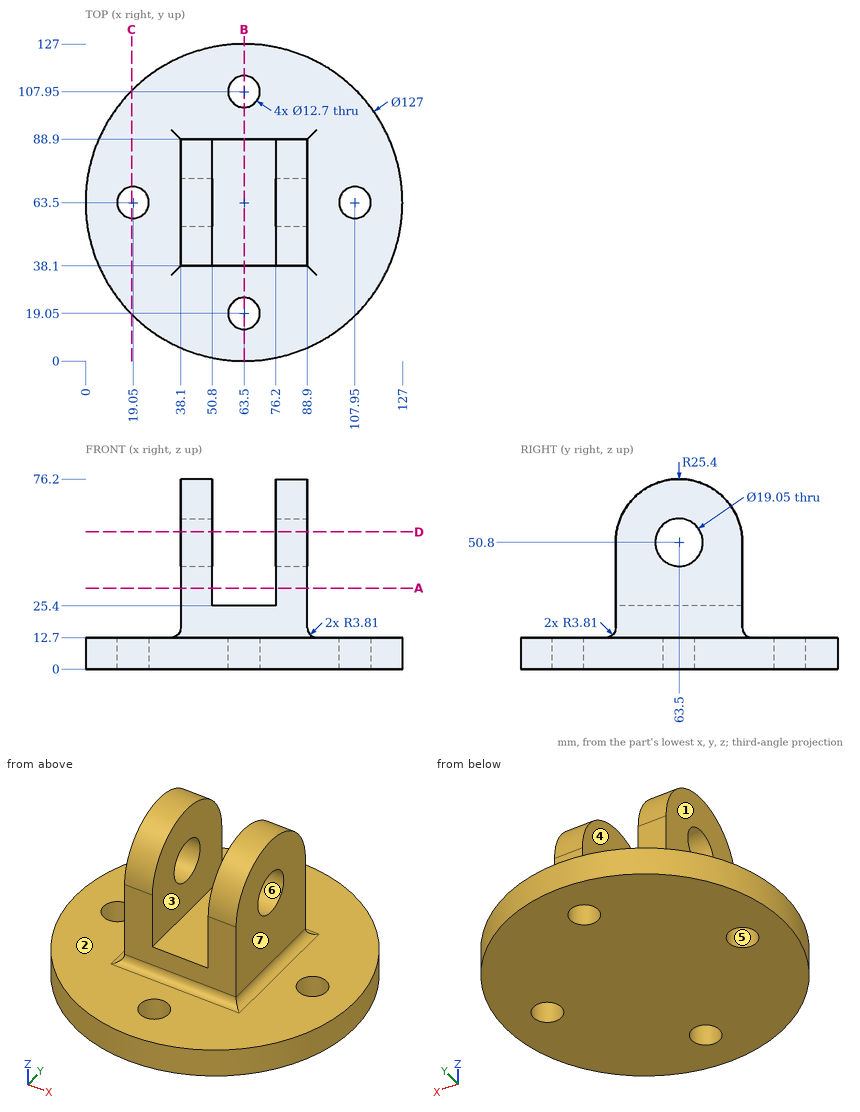
Design review of the part shown in the three views and the two pictorial views. Dimensions are in mm from the part's minimum x, y and z. A direction names the side the tool comes from. Coordinates: 2 decimals unless noted, no trailing zeros. Order: outer loops, then holes, each group sorted by start corner. A loop starts at its lowest first (then second) coordinate and runs counter-clockwise, first axis right, second up.
Item 1: Take a section at C-C, the plane x = 18.5. Write out the cut boundary in (y, z), then the cut area to 3 significant figures.
Item 2: For the marked faces 1, 2 and 3, list the 3-axis set-ups (+Z, -Z, +X, -X, +Y, -Y) from which the entire face can be reached by the end or side of a thin tool; tool diameter is ignored.
Item 3: For line 1 (Y direction, x = 63.5, z = 5); line 2 (Z direction, x = 42.25, y = 63.5) (3 decimals); line 3 (Y direction, x = 41, z = 50), list the stretches that pass through material, from the lowest coordinate up.
Item 4: For pin 1 Ø6 at (x, y) = (79, 94) entering from -Z; pin 2 Ø15 at (y, z) = (58.5, 46.5) entering from +X; pin 3 Ø22 at (y, z) = (63.5, 50.8) entering from -X; pin 4 Ø17 at (x, z) = (64.5, 36.5) entering from -Y, all flat-tipped, find the tip position at first contact; note any pin that passes through.
Item 5: The part is to be moulded in two halves that separate along X. For the marked faces 4, 5, 6 and 7, say which applies: pulls with the +X half, pulls with the -X half, needs draft (parallel to the pull), parting line crosses it, or undercut.
Item 6: Take a section at D-D, the plane z = 55. Write out the cut boundary in (x, y).
Item 7: Take a section at B-B, the plane x = 63.5. Write out the cut boundary in (y, z), then the cut area to 3 significant figures.
Item 8: Take a section at A-A, the plane z = 32.5. Write out the cut boundary in (x, y).
The answers:
1. outline: (18.7, 0) - (57.17, 0) - (57.17, 12.7) - (18.7, 12.7) - close; (69.83, 0) - (108.3, 0) - (108.3, 12.7) - (69.83, 12.7) - close
1. area: 977 mm2
2. face 1: +Z, -X, +Y, -Y
2. face 2: +Z
2. face 3: +Z, +Y, -Y
3. line 1: y = 0 to 12.7, 25.4 to 101.6, 114.3 to 127
3. line 2: z = 0 to 41.275, 60.325 to 76.2
3. line 3: y = 38.1 to 54.01, 72.99 to 88.9
4. pin 1: stops at z = 0
4. pin 2: stops at x = 88.9
4. pin 3: stops at x = 38.1
4. pin 4: passes through
5. face 4: undercut
5. face 5: undercut
5. face 6: needs draft
5. face 7: pulls with the +X half
6. outline: (38.1, 38.45) - (50.8, 38.45) - (50.8, 54.95) - (38.1, 54.95) - close; (38.1, 72.05) - (50.8, 72.05) - (50.8, 88.55) - (38.1, 88.55) - close; (76.2, 38.45) - (88.9, 38.45) - (88.9, 54.95) - (76.2, 54.95) - close; (76.2, 72.05) - (88.9, 72.05) - (88.9, 88.55) - (76.2, 88.55) - close
7. outline: (0, 0) - (12.7, 0) - (12.7, 12.7) - (0, 12.7) - close; (25.4, 0) - (101.6, 0) - (101.6, 12.7) - (92.71, 12.7) arc R3.81 cw to (88.9, 16.51) - (88.9, 25.4) - (38.1, 25.4) - (38.1, 16.51) arc R3.81 cw to (34.29, 12.7) - (25.4, 12.7) - close; (114.3, 0) - (127, 0) - (127, 12.7) - (114.3, 12.7) - close
7. area: 1,940 mm2
8. outline: (38.1, 38.1) - (50.8, 38.1) - (50.8, 88.9) - (38.1, 88.9) - close; (76.2, 38.1) - (88.9, 38.1) - (88.9, 88.9) - (76.2, 88.9) - close
